from build123d import *

# Parameters (mm, degrees)
BOSS_EXTRUDE1_DEPTH = 57
CUT_EXTRUDE1_DEPTH  = 58


with BuildPart() as part:
    # Sketch2 → Boss-Extrude1 (new body)
    with BuildSketch(Plane(origin=(0, 0, 0), x_dir=(0, 0, -1), z_dir=(1, 0, 0))):
        with BuildLine():
            Line((-110.680525015, 0), (-110.680525015, -32.921204516))
            Line((-110.680525015, -32.921204516), (-90.326809139, -50))
            Line((-90.326809139, -50), (47.311208732, -50))
            Line((47.311208732, -50), (63.319474985, -27.968828863))
            Line((63.319474985, -27.968828863), (63.319474985, 109.669189008))
            Line((63.319474985, 109.669189008), (46.240679501, 124))
            Line((46.240679501, 124), (13.319474985, 124))
            Line((13.319474985, 124), (13.319474985, 13.319474985))
            ThreePointArc((13.319474985, 13.319474985), (9.418291084, 3.901183901), (0, 0))
            Line((0, 0), (-110.680525015, 0))
        make_face()
    extrude(amount=BOSS_EXTRUDE1_DEPTH)

    # Sketch3 → Cut-Extrude1 (cut, through all)
    with BuildSketch(Plane(origin=(57, 0, 0), x_dir=(0, 0, -1), z_dir=(1, 0, 0))):
        Polygon((-76.075907073, -45.5), (-76.075907073, -50), (30.330747693, -50), (30.330747693, -45.5), (27.461329109, -42.5), (-73.206488489, -42.5), align=None)
    extrude(amount=-CUT_EXTRUDE1_DEPTH, mode=Mode.SUBTRACT)


solid = part.part
Read the model definition and answer for the solid it produces. Units are mm, in the model's axes. A direction names the side the tool comes from. Round coordinates to 2 decimals unless told otherwise and drop trailing zeros. Write each loop counter-clockwise with the first axis right and the second up, starting at its lowest first coordinate (ties: lowest second). Pieces come first, ordered by that corner, then holes.
Q1. The mould has two halves that part along Z. Classify faces 1 (the face through (28, 0, 55)), 2 (the face through (29, -48, 76.076)), 3 (the face through (28, -16, 110.681)): released by +Z, released by -Z, zero draft, split by the parting line, or undercut.
Values:
face 1: zero draft
face 2: undercut
face 3: released by +Z
Q2. Find section B-B on y = 56. Determine the outline of the cut face in (x, z).
Values:
outline: (0, -63.32) - (57, -63.32) - (57, -13.32) - (0, -13.32) - close
Q3. Find section C-C on z = 80.5. Determine the outline of the cut face in (x, y), and give its area (3 significant figures).
Values:
outline: (0, -50) - (57, -50) - (57, 0) - (0, 0) - close
area: 2,850 mm2
Q4. A tool of negligible diameter and unlimited length cuts with its end or side. For faces 4 (the face through (28.1, -39.14, -55.2)), 5 (the face through (29, -42.5, 22)), 6 (the face through (28, 69, -13.319)), from which of +Z, -Z, +X, -X, +Y, -Y can it reach the whole face along a straight path? Write none if from no direction.
Values:
face 4: -Z, +X, -X, -Y
face 5: +X, -X, -Y
face 6: +Z, +X, -X, +Y
Q5. Find section A-A on x = 22.5. Determine the outline of the cut face in (y, z).
Values:
outline: (-50, -47.31) - (-27.97, -63.32) - (109.67, -63.32) - (124, -46.24) - (124, -13.32) - (13.32, -13.32) arc R13.32 cw to (0, 0) - (0, 110.68) - (-32.92, 110.68) - (-50, 90.33) - (-50, 76.08) - (-45.5, 76.08) - (-42.5, 73.21) - (-42.5, -27.46) - (-45.5, -30.33) - (-50, -30.33) - close
Q6. Flat-ended cylindrical pins translate along their axes: P1, Ø17, axis at x = 19.5, y = 80.5, coming from the +Z side; P2, Ø1.3, axis at x = 27, y = -48.5, coming from the +Z side; P3, Ø12, axis at x = 35, z = 49, coming from the +Y side. Find the tip coordinate at first contact, or state that the pin passes through.
Values:
P1: stops at z = -13.32
P2: stops at z = 92.89
P3: stops at y = 0
Q7. Straight lines are drawn through the part: line 1 (Y direction, x = 17, z = 8.5); line 2 (Z direction, x = 15, y = 42); line 3 (Y direction, x = 6, z = 80). For each, find the intervals that lie inside material, in ascending order.
Values:
line 1: y = -42.5 to 0
line 2: z = -63.32 to -13.32
line 3: y = -50 to 0
